Geometry check sheet. Reference: drawing and pictorial views, mm from the part's lowest x, y, z. A direction names the side the tool comes from. Coordinates: 2 decimals unless noted, no trailing zeros. Write each loop counter-clockwise with the first axis right and the second up, starting at its lowest first coordinate (ties: lowest second). Pieces come first, ordered by that corner, then holes. Notation, with made-up numbers: (-12.5, 56.25) -> (29.5, 56.25) arc R18 ccw to (29.5, 60.25) -> close; hole circle Ø3 at (-35.5, 51). An arc over 180 degrees is marked (long way). Use a Markdown table: item, result.
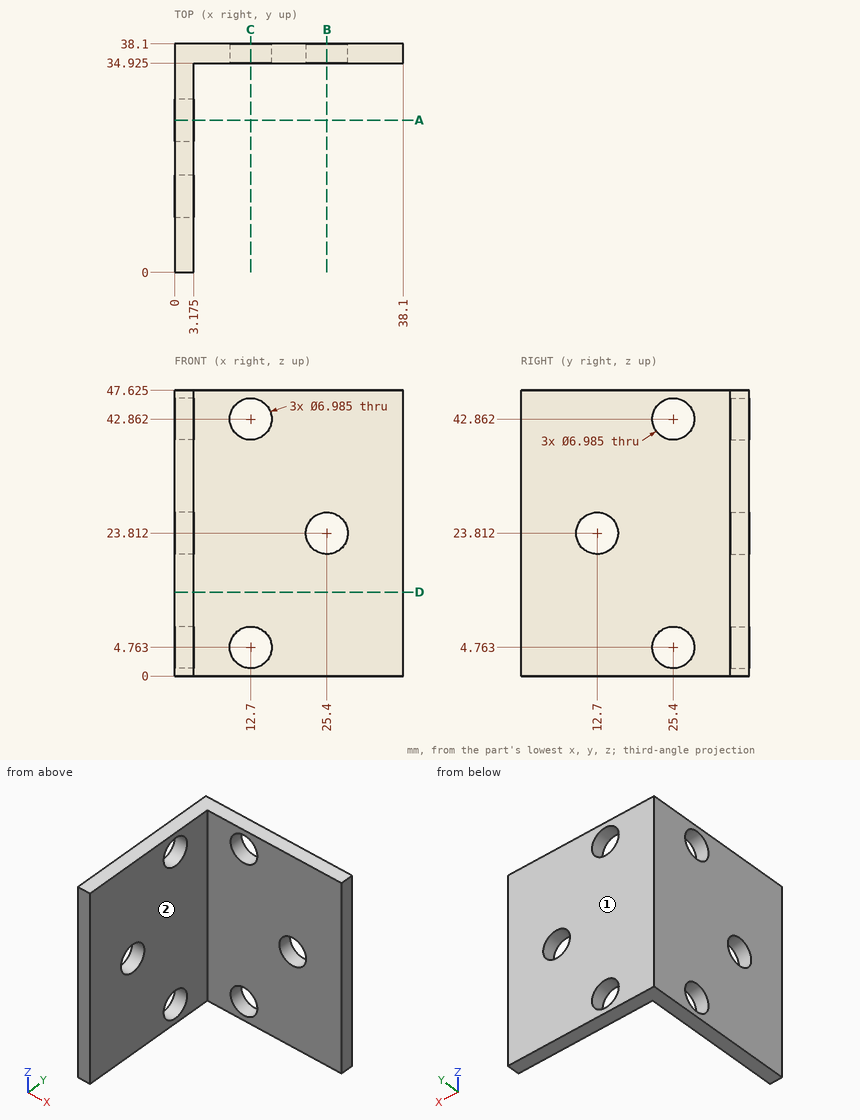
Item 1: Thickness scan on L1, parallel to Z at x = 12.7, y = 37.1 (1 decimal); L2, parallel to Y at x = 22.5, z = 46 (1 decimal); L3, parallel to X at y = 16, z = 18 (1 decimal). Record the ranges inside material, lowest first. Write a range as [from, to].
Answer block:
| item | result |
|---|---|
| L1 | z = [0, 1.3], [8.3, 39.4], [46.4, 47.6] |
| L2 | y = [34.9, 38.1] |
| L3 | x = [0, 3.2] |
Item 2: Section check A-A on y = 25.4. Record the boundary of the cut face in (x, z) (1 decimal).
Answer block:
| item | result |
|---|---|
| outline | (0, 0) -> (3.2, 0) -> (3.2, 1.3) -> (0, 1.3) -> close; (0, 8.3) -> (3.2, 8.3) -> (3.2, 39.4) -> (0, 39.4) -> close; (0, 46.4) -> (3.2, 46.4) -> (3.2, 47.6) -> (0, 47.6) -> close |
Item 3: Tool access check on the marked faces 1 and 2. Record the directions out of +Z, -Z, +X, -X, +Y, -Y that give a thin tool (end or side, any length) a straight path to the whole face; none if there is none.
Answer block:
| item | result |
|---|---|
| face 1 | +Z, -Z, +X, -X, +Y |
| face 2 | +Z, -Z, +X, -Y |
Item 4: Depth check by flat-ended pin: P1, Ø5, axis at y = 16.5, z = 9, coming from the +X side (1 decimal); P2, Ø11, axis at x = 25.4, z = 23.81, coming from the -Y side (1 decimal); P3, Ø5.5, axis at x = 12.7, z = 4.76, coming from the +Y side. Enter the tip coordinate at first touch or a pass-through.
Answer block:
| item | result |
|---|---|
| P1 | stops at x = 3.2 |
| P2 | stops at y = 34.9 |
| P3 | passes through |
Item 5: Section check C-C on x = 12.7. Record the boundary of the cut face in (y, z) (1 decimal).
Answer block:
| item | result |
|---|---|
| outline | (34.9, 0) -> (38.1, 0) -> (38.1, 1.3) -> (34.9, 1.3) -> close; (34.9, 8.3) -> (38.1, 8.3) -> (38.1, 39.4) -> (34.9, 39.4) -> close; (34.9, 46.4) -> (38.1, 46.4) -> (38.1, 47.6) -> (34.9, 47.6) -> close |
Item 6: Section check D-D on z = 14. Record the boundary of the cut face in (x, y) (1 decimal), then the cut area to 3 significant figures.
Answer block:
| item | result |
|---|---|
| outline | (0, 0) -> (3.2, 0) -> (3.2, 34.9) -> (38.1, 34.9) -> (38.1, 38.1) -> (0, 38.1) -> close |
| area | 232 mm^2 |
Item 7: Section check B-B on x = 25.4. Record the boundary of the cut face in (y, z) (1 decimal).
Answer block:
| item | result |
|---|---|
| outline | (34.9, 0) -> (38.1, 0) -> (38.1, 20.3) -> (34.9, 20.3) -> close; (34.9, 27.3) -> (38.1, 27.3) -> (38.1, 47.6) -> (34.9, 47.6) -> close |
